```python
from build123d import *

# Parameters (mm, degrees)
SKETCH1_W           = 264
SKETCH1_H           = 185
SKETCH1_W_2         = 256
SKETCH1_H_2         = 177
BOSS_EXTRUDE4_DEPTH = 75
SKETCH6_W           = 256
SKETCH6_H           = 4
BOSS_EXTRUDE5_DEPTH = 177
SKETCH7_R           = 3
CUT_EXTRUDE1_DEPTH  = 185


with BuildPart() as part:
    # Sketch1 → Boss-Extrude4 (new body)
    with BuildSketch(Plane(origin=(0, 0, 0), x_dir=(1, 0, 0), z_dir=(0, 1, 0))):
        with Locations((1.484105733, 6.470202951)):
            Rectangle(SKETCH1_W, SKETCH1_H)
        with Locations((1.484105733, 6.470202951)):
            Rectangle(SKETCH1_W_2, SKETCH1_H_2, mode=Mode.SUBTRACT)
    extrude(amount=BOSS_EXTRUDE4_DEPTH)

    # Sketch6 → Boss-Extrude5 (add)
    with BuildSketch(Plane.XY.offset(-94.970202951)):
        with Locations((1.484105733, 2)):
            Rectangle(SKETCH6_W, SKETCH6_H)
    extrude(amount=BOSS_EXTRUDE5_DEPTH)

    # Sketch7 → Cut-Extrude1 (cut)
    with BuildSketch(Plane.XY.offset(86.029797049)):
        with Locations((0, 18)):
            Circle(SKETCH7_R)
        with Locations((80, 18)):
            Circle(SKETCH7_R)
    extrude(amount=-CUT_EXTRUDE1_DEPTH, mode=Mode.SUBTRACT)


solid = part.part
```
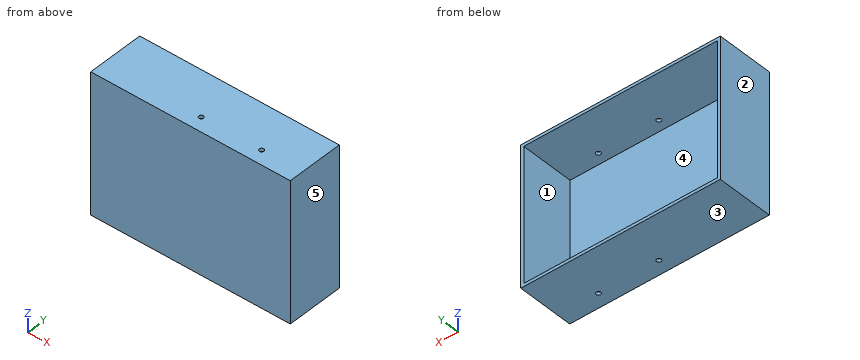
The listing builds one solid part. Answer for the finished solid, in the listing's coordinates (mm). Face numbers are marked on the shaded views. A direction names the side the tool comes from. Coordinates: 2 decimals unless noted, no trailing zeros. Write each loop counter-clockwise with the first axis right and the second up, starting at its lowest first coordinate (ties: lowest second). Pieces come first, ordered by that corner, then holes. Notation, with made-up numbers: (23, 84) - (48, 84) arc R16 cw to (48, 90) - close; hole circle Ø1 at (46, 26.5). An arc over 180 degrees is marked (long way). Return JSON: item names as keys, results as strings. Group by question number.
Q1. Which of the six approach directions +Z, -Z, +X, -X, +Y, -Y give full straight-line access (tool end or side, diameter ignored) to the marked faces 1 and 2?
Q2. The part is cut by section D-D on z = 33. Write down the section's boundary in (x, y).
Q3. Find the intervals of material crossed by line 1 along Z through (x, y) = (2, 45); line 2 along X through (y, z) = (11, 48); line 3 along Y through (x, z) = (80, -96.6), in increasing order. Write a range as [from, to].
Q4. The part is cut by section B-B on x = 0. Write down the section's boundary in (y, z), and give its area (3 significant figures).
Q5. The part is cut by section A-A on y = 18. Write down the section's boundary in (x, z), and give its area (3 significant figures).
Q6. Flat-ended cylindrical pins translate along their axes: pin 1 Ø1 at (x, z) = (37, -75.5) entering from -Y; pin 2 Ø5.5 at (x, y) = (0, 18) entering from -Z; pin 3 Ø1 at (x, z) = (55, -4.5) entering from +Y. Find the tip coordinate at first contact, or state that the pin passes through.
Q7. The part is cut by section C-C on y = 59. Write down the section's boundary in (x, z), and give its area (3 significant figures).
Q8. For a pull along Z with two mould halves and no side action, classify the marked faces 3, 4 and 5 as +Z half, -Z half, draft (parallel to the pull), parting line (faces both ways), or undercut.
Evaluation:
{
 "1": {"face 1": "+Y", "face 2": "+Z, -Z, -X, +Y, -Y"},
 "2": {"outline": "(-130.52, 0) - (133.48, 0) - (133.48, 75) - (129.48, 75) - (129.48, 4) - (-126.52, 4) - (-126.52, 75) - (-130.52, 75) - close"},
 "3": {"line 1": "z = [-98.97, -94.97], [82.03, 86.03]", "line 2": "x = [-130.52, -126.52], [129.48, 133.48]", "line 3": "y = [0, 15], [21, 75]"},
 "4": {"outline": "(0, -98.97) - (15, -98.97) - (15, -94.97) - (4, -94.97) - (4, 82.03) - (15, 82.03) - (15, 86.03) - (0, 86.03) - close; (21, -98.97) - (75, -98.97) - (75, -94.97) - (21, -94.97) - close; (21, 82.03) - (75, 82.03) - (75, 86.03) - (21, 86.03) - close", "area": "1,260 mm2"},
 "5": {"outline": "(-130.52, -98.97) - (-3, -98.97) - (-3, -94.97) - (-126.52, -94.97) - (-126.52, 82.03) - (-3, 82.03) - (-3, 86.03) - (-130.52, 86.03) - close; (3, -98.97) - (77, -98.97) - (77, -94.97) - (3, -94.97) - close; (3, 82.03) - (77, 82.03) - (77, 86.03) - (3, 86.03) - close; (83, -98.97) - (133.48, -98.97) - (133.48, 86.03) - (83, 86.03) - (83, 82.03) - (129.48, 82.03) - (129.48, -94.97) - (83, -94.97) - close", "area": "3,430 mm2"},
 "6": {"pin 1": "stops at y = 0", "pin 2": "passes through", "pin 3": "stops at y = 4"},
 "7": {"outline": "(-130.52, -98.97) - (133.48, -98.97) - (133.48, 86.03) - (-130.52, 86.03) - close; hole (-126.52, -94.97) - (129.48, -94.97) - (129.48, 82.03) - (-126.52, 82.03) - close", "area": "3,530 mm2"},
 "8": {"face 3": "-Z half", "face 4": "undercut", "face 5": "draft"}
}
